The listing builds one solid part. Answer for the finished solid, in the listing's coordinates (mm). A direction names the side the tool comes from. Coordinates: 2 decimals unless noted, no trailing zeros. Loops run counter-clockwise (first coordinate to the right, second up) from the corner with the lowest first, then second, coordinate; pieces in that order, holes last. Notation, with made-up numbers: M -2,73.5 L 4,73.5 A15 cw 4,86.5 Z; hole C -34.75,12 d2. An arc over 180 degrees is marked long. Answer as a JSON object with one key per item and string values. Group by question number.
1. A cutting plane is placed at B-B on x = 5. Give the vertices of the cut face in (y, z), and give its area (3 significant figures).
2. A cutting plane is placed at A-A on y = 11.75. Give the vertices of the cut face in (x, z), and give its area (3 significant figures).
3. For faces 4 (the face through (0.245, 10.897, 1.103)), 5 (the face through (3, 0, 0)), determine the directions among +Z, -Z, +X, -X, +Y, -Y from which every point of the face is accessible in a straight line to the end or side of a thin tool.
4. Straight lines are drawn through the part: L1, parallel to Z at x = 0, y = 10.1; L2, parallel to Z at x = 0, y = 1.5; L3, parallel to X at y = 3.25, z = 2. For each, find the intervals that lie inside material, in ascending order.
5. A cutting plane is placed at D-D on x = -3.5. Give the vertices of the cut face in (y, z), and give its area (3 significant figures).
6. A cutting plane is placed at C-C on y = 2.75. Give the vertices of the cut face in (x, z), and give its area (3 significant figures).
7. Given pin 1 (1.5 mm diameter, centred on x = -3.5, y = 2.5, fed in from +Z); pin 2 (3 mm diameter, centred on x = 0, z = 0, fed in from -Y); pin 3 (3 mm diameter, centred on x = 4, y = 11, fed in from +Z), each flat-ended and moving along its own axis, determine where each tip first touches the part or whether it passes through.
8. Determine the mould class of faces 1 (the face through (-1.38, 6.26, 6.2)), 2 (the face through (1.3, 12.7, -0.1)), 3 (the face through (2.58, 3.04, -0.81)) for opening direction X: released by +X, released by -X, zero draft, split by the parting line, or undercut.
from build123d import *

# Parameters (mm, degrees)
SKETCH1_R                   = 6.35
BOSS_EXTRUDE1_DEPTH         = 12.7
F_4_40_TAPPED_HOLE1_D       = 2.2606
F_4_40_TAPPED_HOLE1_DEPTH   = 3.556
F_4_40_TAPPED_HOLE1_TIP     = 0.679152758
F_1_4_28_TAPPED_HOLE1_D     = 5.4102
F_1_4_28_TAPPED_HOLE1_DEPTH = 6
F_1_4_28_TAPPED_HOLE1_TIP   = 1.625388061


with BuildPart() as part:
    # Sketch1 → Boss-Extrude1 (new body)
    with BuildSketch(Plane(origin=(0, 0, 0), x_dir=(1, 0, 0), z_dir=(0, 1, 0))):
        Circle(SKETCH1_R)
    extrude(amount=BOSS_EXTRUDE1_DEPTH)

    # #4-40 Tapped Hole1
    with Locations(Plane(origin=(0, 12.7, 0), x_dir=(1, 0, 0), z_dir=(0, 1, 0))):
        with Locations((0, 0)):
            Hole(F_4_40_TAPPED_HOLE1_D / 2, depth=F_4_40_TAPPED_HOLE1_DEPTH)
            with Locations((0, 0, -(F_4_40_TAPPED_HOLE1_DEPTH + F_4_40_TAPPED_HOLE1_TIP / 2))):  # 118° drill point
                Cone(0, F_4_40_TAPPED_HOLE1_D / 2, F_4_40_TAPPED_HOLE1_TIP, mode=Mode.SUBTRACT)

    # 1/4-28 Tapped Hole1
    with Locations(Plane(origin=(0, 0, 0), x_dir=(-1, 0, 0), z_dir=(0, -1, 0))):
        with Locations((0, 0)):
            Hole(F_1_4_28_TAPPED_HOLE1_D / 2, depth=F_1_4_28_TAPPED_HOLE1_DEPTH)
            with Locations((0, 0, -(F_1_4_28_TAPPED_HOLE1_DEPTH + F_1_4_28_TAPPED_HOLE1_TIP / 2))):  # 118° drill point
                Cone(0, F_1_4_28_TAPPED_HOLE1_D / 2, F_1_4_28_TAPPED_HOLE1_TIP, mode=Mode.SUBTRACT)


solid = part.part
From the geometry:
{
 "1": {"outline": "M 0,-3.91 L 12.7,-3.91 L 12.7,3.91 L 0,3.91 Z", "area": "99.4 mm²"},
 "2": {"outline": "C 0,0 d12.7; hole C 0,0 d2.26", "area": "123 mm²"},
 "3": {"face 4": "+Y", "face 5": "+Z, -Z, +X, -X, -Y"},
 "4": {"L1": "z = -6.35 to -1.13, 1.13 to 6.35", "L2": "z = -6.35 to -2.71, 2.71 to 6.35", "L3": "x = -6.03 to -1.82, 1.82 to 6.03"},
 "5": {"outline": "M 0,-5.3 L 12.7,-5.3 L 12.7,5.3 L 0,5.3 Z", "area": "135 mm²"},
 "6": {"outline": "C 0,0 d12.7; hole C 0,0 d5.41", "area": "104 mm²"},
 "7": {"pin 1": "stops at z = 5.72", "pin 2": "stops at y = 6.72", "pin 3": "stops at z = 5.84"},
 "8": {"face 1": "split by the parting line", "face 2": "zero draft", "face 3": "undercut"}
}
